```python
from build123d import *

# Parameters (mm, degrees)
F0_W     = 203.2
F0_H     = 63.5
F1_DEPTH = 6.35
F2_R     = 26.035
F3_DEPTH = 12.7
F4_R     = 28.575
F4_R_2   = 26.035
F5_DEPTH = 25.4
F7_DEPTH = 31.75
F8_R     = 2.54


# Not quite as in the source:
# - a feature names something its author has since deleted; it is built from what else it names


with BuildPart() as f1:
    # F0 (on Front) → F1 (new body)
    with BuildSketch(Plane.XZ):
        Rectangle(F0_W, F0_H)
    extrude(amount=F1_DEPTH)

    # F2 (on face) → F3 (cut)
    with BuildSketch(Plane.XZ.offset(6.35)):
        with Locations((-64.8028552532, 0)):
            Circle(F2_R)
        Circle(F2_R)
        with Locations((64.77, 0)):
            Circle(F2_R)
    extrude(amount=-F3_DEPTH, mode=Mode.SUBTRACT)

    # F4 (on face) → F5 (join)
    with BuildSketch(Plane.XZ.offset(6.35)):
        with Locations((-64.8028552532, 0)):
            Circle(F4_R)
        with Locations((-64.8028552532, 0)):
            Circle(F4_R_2, mode=Mode.SUBTRACT)
        Circle(F4_R)
        Circle(F4_R_2, mode=Mode.SUBTRACT)
        with Locations((64.77, 0)):
            Circle(F4_R)
        with Locations((64.77, 0)):
            Circle(F4_R_2, mode=Mode.SUBTRACT)
    extrude(amount=F5_DEPTH)

    # F6 (on Top) → F7 (cut, symmetric)
    with BuildSketch(Plane.XY):
        Polygon((35.6169715524, -20.1309207911), (35.6169715524, -32.004), (95.3069715524, -32.004), align=None)
        Polygon((-29.1554266587, -20.1309207911), (-29.1554266587, -32.004), (30.5345733413, -32.004), align=None)
        Polygon((-93.9486771822, -20.1309207911), (-93.9486771822, -32.004), (-34.2586771822, -32.004), align=None)
    extrude(amount=F7_DEPTH, both=True, mode=Mode.SUBTRACT)

    # F8
    f8_edges = [f1.edges().sort_by_distance(p)[0] for p in [
        (-101.6, -3.175, -31.75),
        (-101.6, -3.175, 31.75),
        (101.6, -3.175, 31.75),
        (101.6, -3.175, -31.75),
    ]]
    fillet(f8_edges, radius=F8_R)


solid = f1.part
```
Read the model definition and answer for the solid it produces. Units are mm, in the model's axes. A direction names the side the tool comes from. Coordinates: 2 decimals unless noted, no trailing zeros. Order: outer loops, then holes, each group sorted by start corner. A loop starts at its lowest first (then second) coordinate and runs counter-clockwise, first axis right, second up. Notation, with made-up numbers: (-6.75, -35.75) - (45.25, -35.75) arc R15 cw to (45.25, -12.75) - close; hole circle Ø6 at (26, 81.5). An arc over 180 degrees is marked (long way). Answer as a JSON object with one key per item and string values. Group by question number.
Item 1: Flat-ended cylindrical pins translate along their axes: P1, Ø4, axis at y = -9, z = -3.5, coming from the -X side; P2, Ø4, axis at x = -20, y = -21, coming from the +Z side; P3, Ø3, axis at y = -17.5, z = 8.5, coming from the -X side. Find the tip coordinate at first contact, or state that the pin passes through.
Item 2: Section D-D (y = -4) is taken. Give the vertices of the cut face in (x, z) (3 decimals), plus the area to 3 significant figures.
Item 3: The mould has two halves that part along Z. Classify faces 1 (the face through (-37.547, -15.997, 8.583)), 2 (the face through (101.6, -3, 0)), 3 (the face through (89.603, -12.316, 7.82)): +Z half, -Z half, draft (parallel to the pull), parting line (faces both ways), or undercut.
Item 4: Consider probe 1 along X at (y, z) = (-6.5, 0) (3 decimals); probe 2 along X at (y, z) = (-25, 14); probe 3 along Z at (x, y) = (65, -4.5). Determine where each line is inside the solid, lowest interval first. Write a range as from..to.
Item 5: Section B-B (x = -85) is taken. Give the vertices of the cut face in (y, z), plus the area to 3 significant figures.
Item 6: A tool of negligible diameter and unlimited length cuts with its end or side. For faces 4 (the face through (52.2, -23.43, 23.15)), 5 (the face through (-1, -3, -31.75)), 6 (the face through (-8, -6.35, -28)), from which of +Z, -Z, +X, -X, +Y, -Y can it reach the whole face along a straight path? Write none if from no direction.
Item 7: Section A-A (y = -13) is taken. Give the vertices of the cut face in (x, z) (3 decimals).
Item 8: Section C-C (z = 0) is taken. State how many separate pieces and enclosed holes the cut face has, plus the area to 3 significant figures.
Results are:
{
 "1": {"P1": "stops at x = -93.34", "P2": "stops at z = 22.19", "P3": "stops at x = -92.51"},
 "2": {"outline": "(-101.6, -29.21) arc R2.54 ccw to (-99.06, -31.75) - (99.06, -31.75) arc R2.54 ccw to (101.6, -29.21) - (101.6, 29.21) arc R2.54 ccw to (99.06, 31.75) - (-99.06, 31.75) arc R2.54 ccw to (-101.6, 29.21) - close; hole circle Ø52.07 at (-64.803, 0); hole circle Ø52.07 at (0, 0); hole circle Ø52.07 at (64.77, 0)", "area": "6,510 mm^2"},
 "3": {"face 1": "parting line", "face 2": "draft", "face 3": "undercut"},
 "4": {"probe 1": "x = -93.378..-90.838, -38.768..-36.228, -28.575..-26.035, 26.035..28.575, 36.195..38.735, 90.805..93.345", "probe 2": "x = -42.85..-39.89, 21.95..24.91, 86.72..89.68", "probe 3": "z = -31.75..-26.03, 26.03..31.75"},
 "5": {"outline": "(-21.91, -20.21) - (-6.35, -20.21) - (-6.35, -31.75) - (0, -31.75) - (0, -16.43) - (-21.91, -16.43) - close; (-21.91, 16.43) - (0, 16.43) - (0, 31.75) - (-6.35, 31.75) - (-6.35, 20.21) - (-21.91, 20.21) - close", "area": "312 mm^2"},
 "6": {"face 4": "+Z, -Z, -Y", "face 5": "-Z, +X, -X, +Y, -Y", "face 6": "-Y"},
 "7": {"outline": "circle Ø57.15 at (-64.803, 0); circle Ø57.15 at (0, 0); circle Ø57.15 at (64.77, 0); hole circle Ø52.07 at (-64.803, 0); hole circle Ø52.07 at (0, 0); hole circle Ø52.07 at (64.77, 0)"},
 "8": {"separate pieces": "4", "enclosed holes": "0", "area": "597 mm^2"}
}
